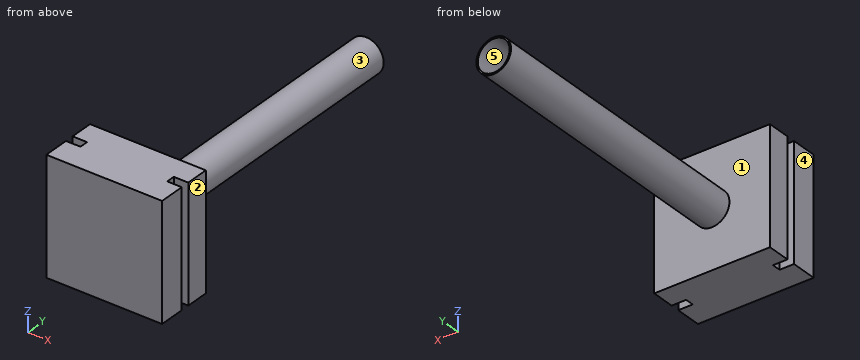
from build123d import *

# Parameters (mm, degrees)
SKETCH1_W           = 400
SKETCH1_H           = 400
BOSS_EXTRUDE1_DEPTH = 200
SKETCH2_R           = 60
SKETCH2_R_2         = 55
BOSS_EXTRUDE2_DEPTH = 1000
SKETCH3_W           = 50
SKETCH3_H           = 30
CUT_EXTRUDE1_DEPTH  = 584


with BuildPart() as part:
    # Sketch1 → Boss-Extrude1 (new body)
    with BuildSketch(Plane(origin=(0, 0, 0), x_dir=(1, 0, 0), z_dir=(0, 1, 0))):
        Rectangle(SKETCH1_W, SKETCH1_H)
    extrude(amount=BOSS_EXTRUDE1_DEPTH)

    # Sketch2 → Boss-Extrude2 (add)
    with BuildSketch(Plane(origin=(0, 200, 0), x_dir=(1, 0, 0), z_dir=(0, 1, 0))):
        Circle(SKETCH2_R)
        Circle(SKETCH2_R_2, mode=Mode.SUBTRACT)
    extrude(amount=BOSS_EXTRUDE2_DEPTH)

    # Sketch3 → Cut-Extrude1 (cut)
    with BuildSketch(Plane(origin=(0, 0, -200), x_dir=(-1, 0, 0), z_dir=(0, 0, -1))):
        with Locations((-175, 105)):
            Rectangle(SKETCH3_W, SKETCH3_H)
        with Locations((175, 105)):
            Rectangle(SKETCH3_W, SKETCH3_H)
    extrude(amount=-CUT_EXTRUDE1_DEPTH, mode=Mode.SUBTRACT)


solid = part.part
Model file for the job. Use its own axes, mm. Face numbers are marked on the shaded views. A direction names the side the tool comes from. Give positions to 0.01 mm unless a question says otherwise; leave off trailing zeros. Order: outer loops, then holes, each group sorted by start corner. A loop starts at its lowest first (then second) coordinate and runs counter-clockwise, first axis right, second up. Notation, with made-up numbers: (3.5, 81.25) - (26.5, 81.25) arc R26 cw to (26.5, 96.25) - close; hole circle Ø5 at (26, 36). An arc over 180 degrees is marked (long way). Return JSON: item names as keys, results as strings.
1) 3-axis set-ups, long thin cutter, end or side, ignore diameter. For the marked faces 1 and 2: which of +Z, -Z, +X, -X, +Y, -Y reach the whole face in a straight line?
Geometry says:
{"face 1": "+Y", "face 2": "+Z, -Z, +X, +Y, -Y"}
2) Cut at A-A, the plane z = 0. Give the cut face in (x, y).
Geometry says:
{"outline": "(-200, 0) - (200, 0) - (200, 90) - (150, 90) - (150, 120) - (200, 120) - (200, 200) - (60, 200) - (60, 1200) - (55, 1200) - (55, 200) - (-55, 200) - (-55, 1200) - (-60, 1200) - (-60, 200) - (-200, 200) - (-200, 120) - (-150, 120) - (-150, 90) - (-200, 90) - close"}
3) Cut at B-B, the plane x = 0. Give the cut face in (y, z), plus the area to 3 significant figures.
Geometry says:
{"outline": "(0, -200) - (200, -200) - (200, -60) - (1200, -60) - (1200, -55) - (200, -55) - (200, 55) - (1200, 55) - (1200, 60) - (200, 60) - (200, 200) - (0, 200) - close", "area": "90,000 mm²"}
4) Flat gauge pins, fed straight in: P1, Ø1, axis at x = -140.5, z = 81, coming from the +Y side; P2, Ø1.5, axis at y = 396, z = -51, coming from the +X side; P3, Ø12, axis at y = 239, z = -48.5, coming from the +X side. Where does each tip first touch, or does it go through?
Geometry says:
{"P1": "y = 200", "P2": "x = 32.79", "P3": "x = 42.35"}
5) Probe line 1 (X direction, y = 621.5, z = 0); line 2 (Y direction, x = 164.5, z = 61). List the from-to ranges inside material, lowest first. Write a range as from..to.
Geometry says:
{"line 1": "-60..-55, 55..60", "line 2": "0..90, 120..200"}
6) Cut at C-C, the plane y = 607. Give the cut face in (x, z), plus the area to 3 significant figures.
Geometry says:
{"outline": "circle Ø120 at (0, 0); hole circle Ø110 at (0, 0)", "area": "1,810 mm²"}
7) Cut at D-D, the plane z = 84. Give the cut face in (x, y).
Geometry says:
{"outline": "(-200, 0) - (200, 0) - (200, 90) - (150, 90) - (150, 120) - (200, 120) - (200, 200) - (-200, 200) - (-200, 120) - (-150, 120) - (-150, 90) - (-200, 90) - close"}
8) Pull direction Z, two halves, no side cores. Call the marked faces 3, 4 and 5: pulls with the +Z half, pulls with the -Z half, needs draft (parallel to the pull), parting line crosses it, or undercut.
Geometry says:
{"face 3": "parting line crosses it", "face 4": "needs draft", "face 5": "undercut"}
